Geometry check sheet. Reference: the model listing, model coordinates, mm. Round coordinates to 2 decimals unless told otherwise and drop trailing zeros. Loops run counter-clockwise (first coordinate to the right, second up) from the corner with the lowest first, then second, coordinate; pieces in that order, holes last. Notation, with made-up numbers: M 19,61.5 L 24,61.5 A16 cw 24,78.5 Z; hole C 89,-17 d7. An arc over 180 degrees is marked long. Use one line per item in the form item = value. Start each with the question number.
1. Cross-section at B-B (z = 41.5). Record the boundary of the cut face in (x, y), then the cut area to 3 significant figures.
2. Cross-section at C-C (y = -3.9). State how many separate pieces and enclosed holes the cut face has, then the cut area to 3 significant figures.
3. Cross-section at A-A (x = 0). Record the boundary of the cut face in (y, z), then the cut area to 3 significant figures.
4. Material ranges on line 1 (Z direction, x = 0, y = -3.4); line 2 (X direction, y = -3.05, z = 8); line 3 (X direction, y = -4.05, z = 5.5), recorded low to high.
5. Cross-section at D-D (z = -13.5). Record the boundary of the cut face in (x, y).
6. Go/stop test with flat-tipped pins: pin 1 (1.4 mm diameter, centred on x = -33, y = -3.5, fed in from +Z); pin 2 (0.5 mm diameter, centred on x = 25, y = -1.5, fed in from +Z); pin 3 (1 mm diameter, centred on y = -4, z = 32, fed in from +X); pin 4 (15 mm diameter, centred on x = 0, z = -36.18, fed in from +Y). Record where each tip stops, or that it passes through.
```python
from build123d import *

# Parameters (mm, degrees)
F0_R     = 50
F0_R_2   = 9.525
F1_DEPTH = 4.9784


with BuildPart() as f1:
    # F0 (on Front) → F1 (new body)
    with BuildSketch(Plane.XZ):
        Circle(F0_R)
        with BuildLine():
            add(Edge.make_bspline(
                [(-13.6288838135, -29.7163466199), (-12.4287970079, -31.0726834254), (-12.4287970079, -33.4598362032)],
                knots=[0, 0, 0, 1, 1, 1], degree=2))
            add(Edge.make_bspline(
                [(-12.4287970079, -33.4598362032), (-12.4287970079, -35.8404785643), (-13.6332240912, -37.204410856)],
                knots=[0, 0, 0, 1, 1, 1], degree=2))
            add(Edge.make_bspline(
                [(-13.6332240912, -37.204410856), (-14.8376511746, -38.5683431476), (-16.9795782579, -38.5683431476)],
                knots=[0, 0, 0, 1, 1, 1], degree=2))
            add(Edge.make_bspline(
                [(-16.9795782579, -38.5683431476), (-19.1692483968, -38.5683431476), (-20.3595695774, -37.2282823837)],
                knots=[0, 0, 0, 1, 1, 1], degree=2))
            add(Edge.make_bspline(
                [(-20.3595695774, -37.2282823837), (-21.5498907579, -35.8882216199), (-21.5498907579, -33.4468153699)],
                knots=[0, 0, 0, 1, 1, 1], degree=2))
            add(Edge.make_bspline(
                [(-21.5498907579, -33.4468153699), (-21.5498907579, -31.0249403699), (-20.356314369, -29.6924750921)],
                knots=[0, 0, 0, 1, 1, 1], degree=2))
            add(Edge.make_bspline(
                [(-20.356314369, -29.6924750921), (-19.1627379801, -28.3600098143), (-16.9665574246, -28.3600098143)],
                knots=[0, 0, 0, 1, 1, 1], degree=2))
            add(Edge.make_bspline(
                [(-16.9665574246, -28.3600098143), (-14.828970619, -28.3600098143), (-13.6288838135, -29.7163466199)],
                knots=[0, 0, 0, 1, 1, 1], degree=2))
        make_face(mode=Mode.SUBTRACT)
        Polygon((-28.6808658119, -28.4316243976), (-34.2082095619, -28.4316243976), (-34.2082095619, -18.5162598143), (-33.0558658119, -18.5162598143), (-33.0558658119, -27.3877875921), (-28.6808658119, -27.3877875921), align=None, mode=Mode.SUBTRACT)
        with Locations((0, -36.1784361303)):
            Circle(F0_R_2, mode=Mode.SUBTRACT)
        with BuildLine():
            Line((32.1758840849, -19.6333272258), (32.1758840849, -29.5486918092))
            Line((32.1758840849, -29.5486918092), (30.8607799182, -29.5486918092))
            Line((30.8607799182, -29.5486918092), (25.4419431127, -21.2283793092))
            Line((25.4419431127, -21.2283793092), (25.3876896404, -21.2283793092))
            add(Edge.make_bspline(
                [(25.3876896404, -21.2283793092), (25.4961965849, -22.6932230592), (25.4961965849, -23.9128411147)],
                knots=[0, 0, 0, 1, 1, 1], degree=2))
            Line((25.4961965849, -23.9128411147), (25.4961965849, -29.5486918092))
            Line((25.4961965849, -29.5486918092), (24.4306583904, -29.5486918092))
            Line((24.4306583904, -29.5486918092), (24.4306583904, -19.6333272258))
            Line((24.4306583904, -19.6333272258), (25.7327417238, -19.6333272258))
            Line((25.7327417238, -19.6333272258), (31.138557696, -27.9210876425))
            Line((31.138557696, -27.9210876425), (31.1928111682, -27.9210876425))
            add(Edge.make_bspline(
                [(31.1928111682, -27.9210876425), (31.1797903349, -27.7387959758), (31.1320472793, -26.7448723647)],
                knots=[0, 0, 0, 1, 1, 1], degree=2))
            add(Edge.make_bspline(
                [(31.1320472793, -26.7448723647), (31.0843042238, -25.7509487536), (31.0973250571, -25.3234313925)],
                knots=[0, 0, 0, 1, 1, 1], degree=2))
            Line((31.0973250571, -25.3234313925), (31.0973250571, -19.6333272258))
            Line((31.0973250571, -19.6333272258), (32.1758840849, -19.6333272258))
        make_face(mode=Mode.SUBTRACT)
        with Locations((-35.2043993771, 0)):
            Circle(F0_R_2, mode=Mode.SUBTRACT)
        with BuildLine():
            add(Edge.make_bspline(
                [(-27.7972958, 29.8964257207), (-26.5158287861, 28.6149587068), (-26.5158287861, 26.3146114846)],
                knots=[0, 0, 0, 1, 1, 1], degree=2))
            add(Edge.make_bspline(
                [(-26.5158287861, 26.3146114846), (-26.5158287861, 23.8601844013), (-27.8482940638, 22.5613562763)],
                knots=[0, 0, 0, 1, 1, 1], degree=2))
            add(Edge.make_bspline(
                [(-27.8482940638, 22.5613562763), (-29.1807593416, 21.2625281513), (-31.6829294805, 21.2625281513)],
                knots=[0, 0, 0, 1, 1, 1], degree=2))
            Line((-31.6829294805, 21.2625281513), (-34.4303253138, 21.2625281513))
            Line((-34.4303253138, 21.2625281513), (-34.4303253138, 31.1778927346))
            Line((-34.4303253138, 31.1778927346), (-31.3921308694, 31.1778927346))
            add(Edge.make_bspline(
                [(-31.3921308694, 31.1778927346), (-29.0787628138, 31.1778927346), (-27.7972958, 29.8964257207)],
                knots=[0, 0, 0, 1, 1, 1], degree=2))
        make_face(mode=Mode.SUBTRACT)
        Polygon((-5.7735026919, 0), (-2.8867513459, 5), (2.8867513459, 5), (5.7735026919, 0), (2.8867513459, -5), (-2.8867513459, -5), align=None, mode=Mode.SUBTRACT)
        with Locations((36.8741750717, 0)):
            Circle(F0_R_2, mode=Mode.SUBTRACT)
        with Locations((0, 37.8482080996)):
            Circle(F0_R_2, mode=Mode.SUBTRACT)
        Polygon((24.0917380744, 33.7066756686), (26.7176061299, 28.7479083074), (29.3608352966, 33.7066756686), (30.6086651577, 33.7066756686), (27.2992033522, 27.6367971963), (27.2992033522, 23.7913110852), (26.1338387688, 23.7913110852), (26.1338387688, 27.5825437241), (22.8308873799, 33.7066756686), align=None, mode=Mode.SUBTRACT)
    extrude(amount=F1_DEPTH)


solid = f1.part
```
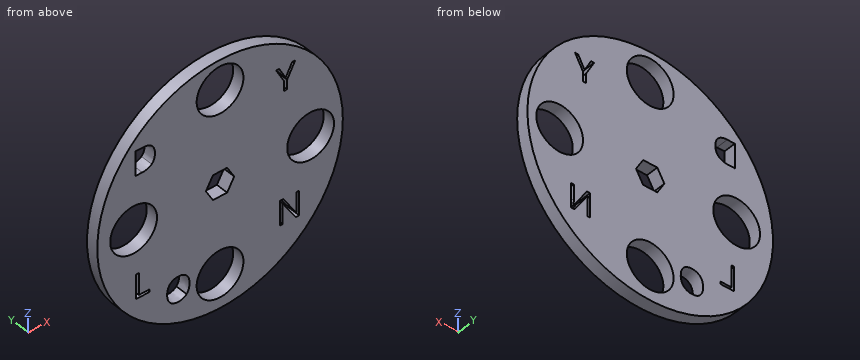
Reported:
q1.outline = M -27.89,-4.98 L -8.8,-4.98 L -8.8,0 L -27.89,0 Z; M 8.8,-4.98 L 27.89,-4.98 L 27.89,0 L 8.8,0 Z
q1.area = 190 mm²
q2.separate_pieces = 1
q2.enclosed_holes = 10
q2.area = 6,410 mm²
q3.outline = M -4.98,-50 L 0,-50 L 0,-45.7 L -4.98,-45.7 Z; M -4.98,-26.65 L 0,-26.65 L 0,-5 L -4.98,-5 Z; M -4.98,5 L 0,5 L 0,28.32 L -4.98,28.32 Z; M -4.98,47.37 L 0,47.37 L 0,50 L -4.98,50 Z
q3.area = 258 mm²
q4.line_1 = -50 to -45.7, -26.65 to -5, 5 to 28.32, 47.37 to 50
q4.line_2 = -49.36 to -40.37, -30.03 to 31.7, 42.04 to 49.36
q4.line_3 = -49.7 to -42.98, -27.43 to 29.1, 44.65 to 49.7
q5.outline = M -48.14,-4.98 L 48.14,-4.98 L 48.14,0 L -48.14,0 Z
q6.pin_1 = 38.17
q6.pin_2 = 43.44
q6.pin_3 = 38.83
q6.pin_4 = through
